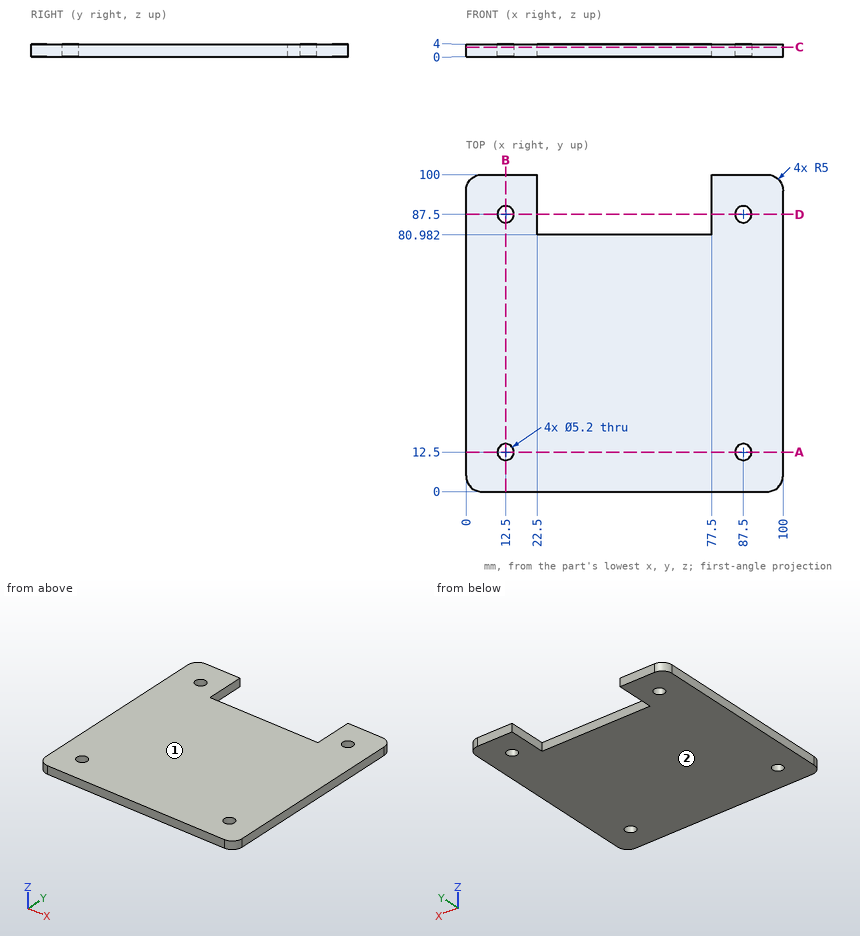
The figure shows three views and two pictorial views of one solid part (mm, origin at its lowest corner). Answer the questions. Coordinates: 2 decimals unless noted, no trailing zeros. Write each loop counter-clockwise with the first axis right and the second up, starting at its lowest first coordinate (ties: lowest second). Pieces come first, ordered by that corner, then holes. Notation, with made-up numbers: (-26, 65) -> (-5, 65) arc R29 cw to (-5, 96) -> close; hole circle Ø11 at (-22, 46). An arc over 180 degrees is marked (long way). Return JSON: item names as keys, results as strings.
1. A cutting plane is placed at C-C (z = 3.05). Determine the outline of the cut face in (x, y), and give its area (3 significant figures).
Found:
{"outline": "(0, 5) arc R5 ccw to (5, 0) -> (95, 0) arc R5 ccw to (100, 5) -> (100, 95) arc R5 ccw to (95, 100) -> (77.5, 100) -> (77.5, 80.98) -> (22.5, 80.98) -> (22.5, 100) -> (5, 100) arc R5 ccw to (0, 95) -> close; hole circle Ø5.2 at (12.5, 12.5); hole circle Ø5.2 at (12.5, 87.5); hole circle Ø5.2 at (87.5, 12.5); hole circle Ø5.2 at (87.5, 87.5)", "area": "8,850 mm2"}
2. This flat-tipped pin is pushed along its axis until it touches: P1, Ø4, axis at x = 12.5, y = 12.5, coming from the +Z side. Where does it stop, or does it pass through?
Found:
{"P1": "through"}
3. A cutting plane is placed at A-A (y = 12.5). Determine the outline of the cut face in (x, z).
Found:
{"outline": "(0, 0) -> (9.9, 0) -> (9.9, 4) -> (0, 4) -> close; (15.1, 0) -> (84.9, 0) -> (84.9, 4) -> (15.1, 4) -> close; (90.1, 0) -> (100, 0) -> (100, 4) -> (90.1, 4) -> close"}
4. Determine the mould class of the marked faces 1 and 2 for opening direction Z: pulls with the +Z half, pulls with the -Z half, needs draft (parallel to the pull), parting line crosses it, or undercut.
Found:
{"face 1": "pulls with the +Z half", "face 2": "pulls with the -Z half"}
5. A cutting plane is placed at D-D (y = 87.5). Determine the outline of the cut face in (x, z).
Found:
{"outline": "(0, 0) -> (9.9, 0) -> (9.9, 4) -> (0, 4) -> close; (15.1, 0) -> (22.5, 0) -> (22.5, 4) -> (15.1, 4) -> close; (77.5, 0) -> (84.9, 0) -> (84.9, 4) -> (77.5, 4) -> close; (90.1, 0) -> (100, 0) -> (100, 4) -> (90.1, 4) -> close"}
6. Find the intervals of material crossed by line 1 along Y through (x, z) = (87.5, 1.9); line 2 along X through (y, z) = (87.5, 1.7); line 3 along Y through (x, z) = (86, 2.3), in increasing order. Write a range as from..to.
Found:
{"line 1": "0..9.9, 15.1..84.9, 90.1..100", "line 2": "0..9.9, 15.1..22.5, 77.5..84.9, 90.1..100", "line 3": "0..10.38, 14.62..85.38, 89.62..100"}
